The listing builds one solid part. Answer for the finished solid, in the listing's coordinates (mm). Face numbers are marked on the shaded views. A direction names the side the tool comes from. Give positions to 0.01 mm unless a question says otherwise; leave off trailing zeros. Order: outer loops, then holes, each group sorted by start corner. A loop starts at its lowest first (then second) coordinate and runs counter-clockwise, first axis right, second up. Notation, with made-up numbers: (-12, -5) - (-5, -5) arc R11 cw to (-5, 15) - close; hole circle Ø5 at (8.5, 79.5). An arc over 180 degrees is marked (long way). Answer in a Markdown table with one row per item. Add a question column.
Autodesk Inventor part; units mm, degrees
ref_plane "YZ Plane" through (0, 0, 0) normal (1, 0, 0) x (0, 1, 0)
ref_plane "XZ Plane" through (0, 0, 0) normal (0, 1, 0) x (-1, 0, 0)
ref_plane "XY Plane" through (0, 0, 0) normal (0, 0, 1) x (1, 0, 0)
sketch "Эскиз1" plane through (0, 0, 0) normal (0, 0, 1) x (1, 0, 0)
  line L0 (7, -11) -> (-7, -11)
  line L1 (-7, -11) -> (-7, 11)
  line L2 (-7, 11) -> (7, 11)
  line L3 (7, 11) -> (7, -11)
  line L4 (7, -11) -> (-7, 11) construction
  line L5 (-7, -11) -> (7, 11) construction
  point P0 (0, 0)
  dimension "d0" = 14
  dimension "d1" = 22
extrude "Выдавливание1" add sketch "Эскиз1" along normal blind 20
sketch "Эскиз2" plane through (0, 0, 20) normal (0, 0, 1) x (1, 0, 0)
  line L0 (7, 11) -> (-7, 11)
  line L1 (-3.5, 11) -> (3.5, 11)
  line L2 (3.5, 11) -> (3.5, -9)
  line L3 (3.5, -9) -> (-3.5, -9)
  line L4 (-3.5, -9) -> (-3.5, 11)
  point P0 (0, 0)
  dimension "d4" = 20
  dimension "d5" = 7
  dimension "d6" = 3.5
extrude "Выдавливание2" cut sketch "Эскиз2" against normal blind 18
sketch "Эскиз3" plane through (0, 0, 20) normal (0, 0, 1) x (1, 0, 0)
  line L0 (3.5, -9) -> (-3.5, -9)
  line L1 (-3.5, -9) -> (-5.5, -9)
  line L2 (-5.5, -9) -> (-5.5, -5)
  line L3 (-5.5, -5) -> (-3.5, -5)
  line L4 (-3.5, -5) -> (-3.5, -9)
  point P0 (0, 0)
  dimension "d9" = 2
  dimension "d10" = 4
extrude "Выдавливание3" cut sketch "Эскиз3" against normal blind 20
properties part number "karmashek"
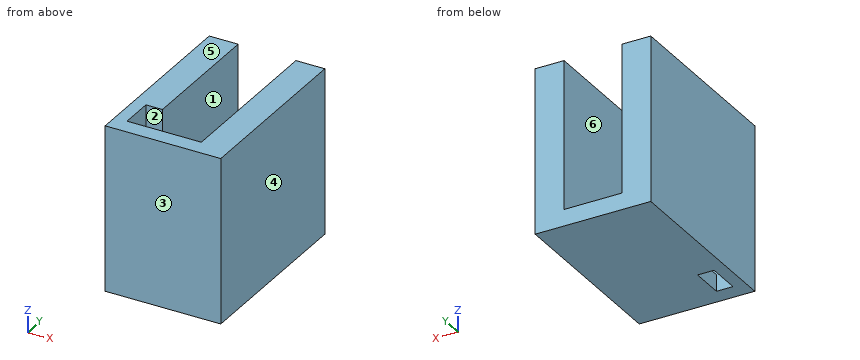
(1) Straight lines are drawn through the part: line 1 (Y direction, x = -5, z = 1.75); line 2 (X direction, y = 8, z = 11.75); line 3 (X direction, y = -8, z = 9.75). For each, find the intervals that lie inside material, in ascending order.
(2) The mould has two halves that part along X. Classify the marked faces 4, 5 and 6: +X half, -X half, draft (parallel to the pull), parting line (faces both ways), or undercut.
(3) Find section A-A, the plane y = -7.5. Write down the section's boundary in (x, z), plus the area to 3 significant figures.
(4) For the marked faces 1, 2 and 3, determine the directions among +Z, -Z, +X, -X, +Y, -Y from which every point of the face is accessible in a straight line to the end or side of a thin tool.
(5) Find section D-D, the plane x = 1.5. Write down the section's boundary in (y, z), plus the area to 3 significant figures.
(6) Each of these flat-tipped pins is pushed along its axis until it touches: P1, Ø5, axis at x = 0, y = 7.5, coming from the -Z side; P2, Ø3.5, axis at x = 0, y = 0.5, coming from the +Z side. Where does it stop, or does it pass through?
(7) Find section C-C, the plane z = 18.75. Write down the section's boundary in (x, y).
(8) Find section B-B, the plane y = 5.5. Write down the section's boundary in (x, z), plus the area to 3 significant figures.
Answer key:
| question | item | result |
|---|---|---|
| 1 | line 1 | -11 to -9, -5 to 11 |
| 1 | line 2 | -7 to -3.5, 3.5 to 7 |
| 1 | line 3 | -7 to -5.5, 3.5 to 7 |
| 2 | face 4 | +X half |
| 2 | face 5 | draft |
| 2 | face 6 | undercut |
| 3 | outline | (-7, 0) - (-5.5, 0) - (-5.5, 20) - (-7, 20) - close; (-3.5, 0) - (7, 0) - (7, 20) - (3.5, 20) - (3.5, 2) - (-3.5, 2) - close |
| 3 | area | 114 mm² |
| 4 | face 1 | +Z, +Y |
| 4 | face 2 | +Z, -Z |
| 4 | face 3 | +Z, -Z, +X, -X, -Y |
| 5 | outline | (-11, 0) - (11, 0) - (11, 2) - (-9, 2) - (-9, 20) - (-11, 20) - close |
| 5 | area | 80.0 mm² |
| 6 | P1 | z = 0 |
| 6 | P2 | z = 2 |
| 7 | outline | (-7, -11) - (7, -11) - (7, 11) - (3.5, 11) - (3.5, -9) - (-5.5, -9) - (-5.5, -5) - (-3.5, -5) - (-3.5, 11) - (-7, 11) - close |
| 8 | outline | (-7, 0) - (7, 0) - (7, 20) - (3.5, 20) - (3.5, 2) - (-3.5, 2) - (-3.5, 20) - (-7, 20) - close |
| 8 | area | 154 mm² |
